Here's the drawing with two shaded views (mm, measured from the low corner). I have some questions. Give positions to 0.01 mm unless a question says otherwise; leave off trailing zeros. Write each loop counter-clockwise with the first axis right and the second up, starting at its lowest first coordinate (ties: lowest second). Pieces come first, ordered by that corner, then holes. Notation, with made-up numbers: (53, 65.25) -> (65, 65.25) arc R13 ccw to (65, 90.25) -> close; hole circle Ø5 at (44.5, 75.5). An arc over 180 degrees is marked (long way). One line per item, written item: value.
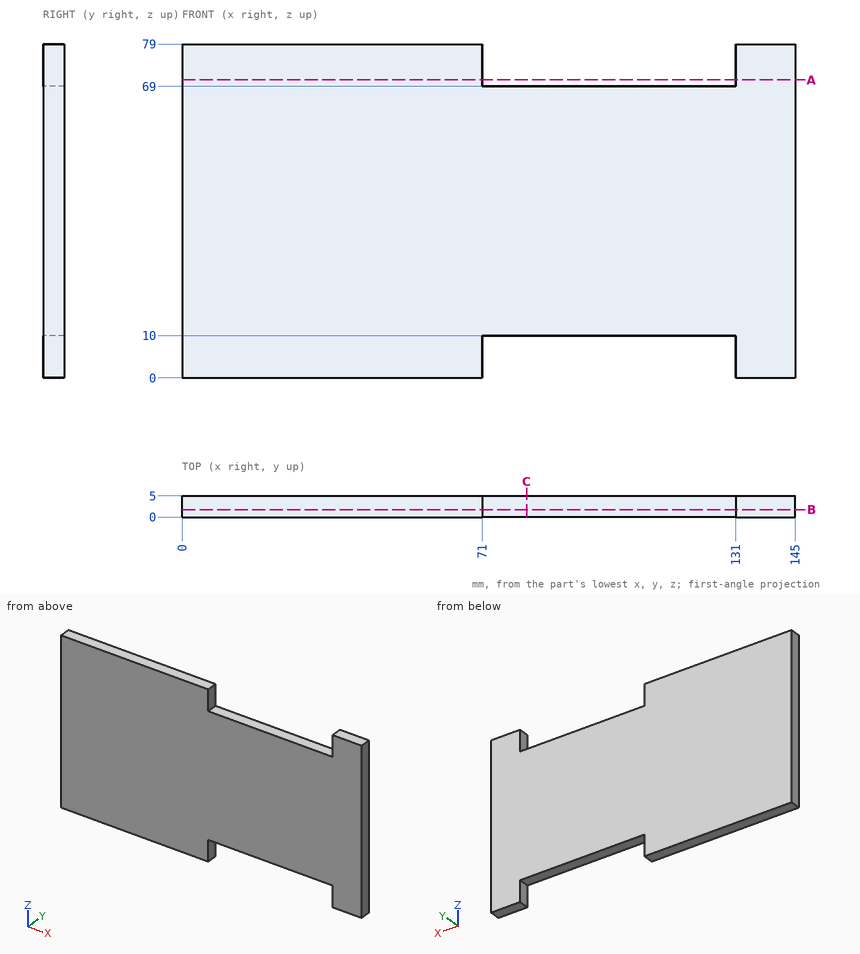
1) If we section it at A-A (z = 70.5): Write out the boundary of the cut face in (x, y).
Answer list:
outline: (0, 0) -> (71, 0) -> (71, 5) -> (0, 5) -> close; (131, 0) -> (145, 0) -> (145, 5) -> (131, 5) -> close
2) Will this pin go through, and if not, where does the flat tip stop? pin 1 (2.5 mm diameter, centred on x = 92, y = 3, fed in from +Z).
Answer list:
pin 1: stops at z = 69
3) I need wall thicknesses on L1, parallel to X at y = 3.15, z = 73.5; L2, parallel to Z at x = 105, y = 3.05. Which ranges of each line are inside material? Lowest first, please.
Answer list:
L1: x = 0 to 71, 131 to 145
L2: z = 10 to 69
4) If we section it at B-B (y = 1.75): Write out the boundary of the cut face in (x, z).
Answer list:
outline: (0, 0) -> (71, 0) -> (71, 10) -> (131, 10) -> (131, 0) -> (145, 0) -> (145, 79) -> (131, 79) -> (131, 69) -> (71, 69) -> (71, 79) -> (0, 79) -> close
5) If we section it at C-C (x = 81.5): Write out the boundary of the cut face in (y, z), and give its area (3 significant figures).
Answer list:
outline: (0, 10) -> (5, 10) -> (5, 69) -> (0, 69) -> close
area: 295 mm^2
